Input: part model. Units: mm. Frame: model coordinates. Coordinates: 2 decimals unless noted, no trailing zeros. Write each loop counter-clockwise with the first axis right and the second up, starting at its lowest first coordinate (ties: lowest second). Pieces come first, ordered by that corner, then holes. Notation, with made-up numbers: (7, 4) - (26, 4) arc R15 cw to (26, 9) - close; hole circle Ø6 at (78.25, 27.5). An arc over 180 degrees is marked (long way). One line per question, with ' | ' between items. Start each with the question number.
1) Section query A-A on z = 216.5. Return loops of the section in (x, y).
2) Section query C-C on y = -0.4. Give the number of separate pieces and of enclosed holes in the cut face, and give its area (3 significant figures).
3) Section query B-B on x = -7838.5. Return loops of the section in (y, z), and give its area (3 significant figures).
4) Line query: line 1 (Z direction, x = -7729.5, y = -0.45); line 2 (Z direction, x = -7732.5, y = -1.35); line 3 (Z direction, x = -7816, y = -0.5). Output: solid intervals per line, ascending.
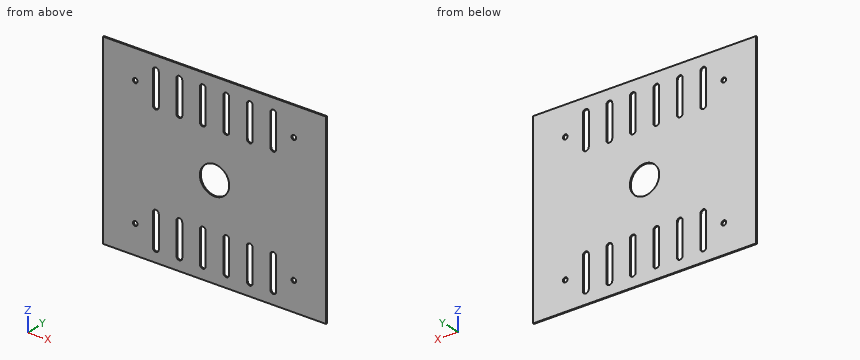
```python
from build123d import *

# Parameters (mm, degrees)
F0_W     = 380
F0_H     = 320
F0_R     = 4
F0_R_2   = 25
F1_DEPTH = 2


with BuildPart() as f1:
    # F0 (on Front) → F1 (new body)
    with BuildSketch(Plane.XZ):
        with Locations((-7832.275127, 205.356488)):
            Rectangle(F0_W, F0_H)
        with Locations((-7967.275127, 94.752941)):
            Circle(F0_R, mode=Mode.SUBTRACT)
        with BuildLine():
            ThreePointArc((-7932.275127, 127.252941), (-7928.739593, 125.788475), (-7927.275127, 122.252941))
            Line((-7927.275127, 122.252941), (-7927.275127, 67.252941))
            ThreePointArc((-7927.275127, 67.252941), (-7928.739593, 63.717407), (-7932.275127, 62.252941))
            ThreePointArc((-7932.275127, 62.252941), (-7935.810661, 63.717407), (-7937.275127, 67.252941))
            Line((-7937.275127, 67.252941), (-7937.275127, 122.252941))
            ThreePointArc((-7937.275127, 122.252941), (-7935.810661, 125.788475), (-7932.275127, 127.252941))
        make_face(mode=Mode.SUBTRACT)
        with BuildLine():
            ThreePointArc((-7892.275127, 127.252941), (-7888.739593, 125.788475), (-7887.275127, 122.252941))
            Line((-7887.275127, 122.252941), (-7887.275127, 67.252941))
            ThreePointArc((-7887.275127, 67.252941), (-7888.739593, 63.717407), (-7892.275127, 62.252941))
            ThreePointArc((-7892.275127, 62.252941), (-7895.810661, 63.717407), (-7897.275127, 67.252941))
            Line((-7897.275127, 67.252941), (-7897.275127, 122.252941))
            ThreePointArc((-7897.275127, 122.252941), (-7895.810661, 125.788475), (-7892.275127, 127.252941))
        make_face(mode=Mode.SUBTRACT)
        with BuildLine():
            ThreePointArc((-7852.275127, 127.252941), (-7848.739593, 125.788475), (-7847.275127, 122.252941))
            Line((-7847.275127, 122.252941), (-7847.275127, 67.252941))
            ThreePointArc((-7847.275127, 67.252941), (-7848.739593, 63.717407), (-7852.275127, 62.252941))
            ThreePointArc((-7852.275127, 62.252941), (-7855.810661, 63.717407), (-7857.275127, 67.252941))
            Line((-7857.275127, 67.252941), (-7857.275127, 122.252941))
            ThreePointArc((-7857.275127, 122.252941), (-7855.810661, 125.788475), (-7852.275127, 127.252941))
        make_face(mode=Mode.SUBTRACT)
        with BuildLine():
            ThreePointArc((-7812.275127, 127.252941), (-7808.739593, 125.788475), (-7807.275127, 122.252941))
            Line((-7807.275127, 122.252941), (-7807.275127, 67.252941))
            ThreePointArc((-7807.275127, 67.252941), (-7808.739593, 63.717407), (-7812.275127, 62.252941))
            ThreePointArc((-7812.275127, 62.252941), (-7815.810661, 63.717407), (-7817.275127, 67.252941))
            Line((-7817.275127, 67.252941), (-7817.275127, 122.252941))
            ThreePointArc((-7817.275127, 122.252941), (-7815.810661, 125.788475), (-7812.275127, 127.252941))
        make_face(mode=Mode.SUBTRACT)
        with BuildLine():
            ThreePointArc((-7772.275127, 127.252941), (-7768.739593, 125.788475), (-7767.275127, 122.252941))
            Line((-7767.275127, 122.252941), (-7767.275127, 67.252941))
            ThreePointArc((-7767.275127, 67.252941), (-7768.739593, 63.717407), (-7772.275127, 62.252941))
            ThreePointArc((-7772.275127, 62.252941), (-7775.810661, 63.717407), (-7777.275127, 67.252941))
            Line((-7777.275127, 67.252941), (-7777.275127, 122.252941))
            ThreePointArc((-7777.275127, 122.252941), (-7775.810661, 125.788475), (-7772.275127, 127.252941))
        make_face(mode=Mode.SUBTRACT)
        with BuildLine():
            ThreePointArc((-7732.275127, 127.252941), (-7728.739593, 125.788475), (-7727.275127, 122.252941))
            Line((-7727.275127, 122.252941), (-7727.275127, 67.252941))
            ThreePointArc((-7727.275127, 67.252941), (-7728.739593, 63.717407), (-7732.275127, 62.252941))
            ThreePointArc((-7732.275127, 62.252941), (-7735.810661, 63.717407), (-7737.275127, 67.252941))
            Line((-7737.275127, 67.252941), (-7737.275127, 122.252941))
            ThreePointArc((-7737.275127, 122.252941), (-7735.810661, 125.788475), (-7732.275127, 127.252941))
        make_face(mode=Mode.SUBTRACT)
        with Locations((-7697.275127, 94.752941)):
            Circle(F0_R, mode=Mode.SUBTRACT)
        with Locations((-7832.275127, 205.356488)):
            Circle(F0_R_2, mode=Mode.SUBTRACT)
        with Locations((-7967.275127, 315.356488)):
            Circle(F0_R, mode=Mode.SUBTRACT)
        with BuildLine():
            ThreePointArc((-7932.275127, 347.008945), (-7928.739593, 345.544479), (-7927.275127, 342.008945))
            Line((-7927.275127, 342.008945), (-7927.275127, 287.008945))
            ThreePointArc((-7927.275127, 287.008945), (-7928.739593, 283.473411), (-7932.275127, 282.008945))
            ThreePointArc((-7932.275127, 282.008945), (-7935.810661, 283.473411), (-7937.275127, 287.008945))
            Line((-7937.275127, 287.008945), (-7937.275127, 342.008945))
            ThreePointArc((-7937.275127, 342.008945), (-7935.810661, 345.544479), (-7932.275127, 347.008945))
        make_face(mode=Mode.SUBTRACT)
        with BuildLine():
            ThreePointArc((-7892.275127, 347.008945), (-7888.739593, 345.544479), (-7887.275127, 342.008945))
            Line((-7887.275127, 342.008945), (-7887.275127, 287.008945))
            ThreePointArc((-7887.275127, 287.008945), (-7888.739593, 283.473411), (-7892.275127, 282.008945))
            ThreePointArc((-7892.275127, 282.008945), (-7895.810661, 283.473411), (-7897.275127, 287.008945))
            Line((-7897.275127, 287.008945), (-7897.275127, 342.008945))
            ThreePointArc((-7897.275127, 342.008945), (-7895.810661, 345.544479), (-7892.275127, 347.008945))
        make_face(mode=Mode.SUBTRACT)
        with BuildLine():
            ThreePointArc((-7852.275127, 347.008945), (-7848.739593, 345.544479), (-7847.275127, 342.008945))
            Line((-7847.275127, 342.008945), (-7847.275127, 287.008945))
            ThreePointArc((-7847.275127, 287.008945), (-7848.739593, 283.473411), (-7852.275127, 282.008945))
            ThreePointArc((-7852.275127, 282.008945), (-7855.810661, 283.473411), (-7857.275127, 287.008945))
            Line((-7857.275127, 287.008945), (-7857.275127, 342.008945))
            ThreePointArc((-7857.275127, 342.008945), (-7855.810661, 345.544479), (-7852.275127, 347.008945))
        make_face(mode=Mode.SUBTRACT)
        with BuildLine():
            ThreePointArc((-7812.275127, 347.008945), (-7808.739593, 345.544479), (-7807.275127, 342.008945))
            Line((-7807.275127, 342.008945), (-7807.275127, 287.008945))
            ThreePointArc((-7807.275127, 287.008945), (-7808.739593, 283.473411), (-7812.275127, 282.008945))
            ThreePointArc((-7812.275127, 282.008945), (-7815.810661, 283.473411), (-7817.275127, 287.008945))
            Line((-7817.275127, 287.008945), (-7817.275127, 342.008945))
            ThreePointArc((-7817.275127, 342.008945), (-7815.810661, 345.544479), (-7812.275127, 347.008945))
        make_face(mode=Mode.SUBTRACT)
        with BuildLine():
            ThreePointArc((-7772.275127, 347.008945), (-7768.739593, 345.544479), (-7767.275127, 342.008945))
            Line((-7767.275127, 342.008945), (-7767.275127, 287.008945))
            ThreePointArc((-7767.275127, 287.008945), (-7768.739593, 283.473411), (-7772.275127, 282.008945))
            ThreePointArc((-7772.275127, 282.008945), (-7775.810661, 283.473411), (-7777.275127, 287.008945))
            Line((-7777.275127, 287.008945), (-7777.275127, 342.008945))
            ThreePointArc((-7777.275127, 342.008945), (-7775.810661, 345.544479), (-7772.275127, 347.008945))
        make_face(mode=Mode.SUBTRACT)
        with BuildLine():
            ThreePointArc((-7732.275127, 347.008945), (-7728.739593, 345.544479), (-7727.275127, 342.008945))
            Line((-7727.275127, 342.008945), (-7727.275127, 287.008945))
            ThreePointArc((-7727.275127, 287.008945), (-7728.739593, 283.473411), (-7732.275127, 282.008945))
            ThreePointArc((-7732.275127, 282.008945), (-7735.810661, 283.473411), (-7737.275127, 287.008945))
            Line((-7737.275127, 287.008945), (-7737.275127, 342.008945))
            ThreePointArc((-7737.275127, 342.008945), (-7735.810661, 345.544479), (-7732.275127, 347.008945))
        make_face(mode=Mode.SUBTRACT)
        with Locations((-7697.275127, 315.356488)):
            Circle(F0_R, mode=Mode.SUBTRACT)
    extrude(amount=F1_DEPTH)


solid = f1.part
```
Answer key:
1) outline: (-8022.28, -2) - (-7854.65, -2) - (-7854.65, 0) - (-8022.28, 0) - close; (-7809.9, -2) - (-7642.28, -2) - (-7642.28, 0) - (-7809.9, 0) - close
2) separate pieces: 1 | enclosed holes: 17 | area: 112,000 mm²
3) outline: (-2, 45.36) - (0, 45.36) - (0, 181.14) - (-2, 181.14) - close; (-2, 229.57) - (0, 229.57) - (0, 365.36) - (-2, 365.36) - close | area: 543 mm²
4) line 1: 45.36 to 63.09, 126.41 to 282.85, 346.17 to 365.36 | line 2: 45.36 to 62.26, 127.25 to 282.01, 347 to 365.36 | line 3: 45.36 to 63.92, 125.59 to 186.38, 224.33 to 283.67, 345.34 to 365.36
